from build123d import *

# Parameters (mm, degrees)
F0_W      = 50.8
F0_H      = 31.75
F1_DEPTH  = 31.75
F3_DEPTH  = 50.8
F5_DEPTH  = 50.8
F7_DEPTH  = 25.4
F8_W      = 12.7
F8_H      = 16.2741773874
F9_DEPTH  = 19.05
F11_DEPTH = 25.4


with BuildPart() as f1:
    # F0 (on Front) → F1 (new body)
    with BuildSketch(Plane.XZ):
        with Locations((25.4, 15.875)):
            Rectangle(F0_W, F0_H)
    extrude(amount=F1_DEPTH)

    # F2 (on face) → F3 (cut)
    with BuildSketch(Plane.YZ.offset(50.8)):
        Polygon((-31.75, 31.75), (-31.75, 12.7), (-15.875, 31.75), align=None)
    extrude(amount=-F3_DEPTH, mode=Mode.SUBTRACT)

    # F4 (on face) → F5 (cut)
    with BuildSketch(Plane.YZ.offset(50.8)):
        Polygon((-15.875, 31.75), (-31.75, 12.7), (-15.4758226126, 12.7), align=None)
    extrude(amount=-F5_DEPTH, mode=Mode.SUBTRACT)

    # F6 (on face) → F7 (cut)
    with BuildSketch(Plane(origin=(0, -15.2030290354, -0.3185672131), x_dir=(1, 0, 0), z_dir=(0, -0.9997805332, -0.0209495948))):
        Polygon((38.1, 32.0756067453), (50.8, 13.0214249842), (50.8, 32.0756067453), align=None)
    extrude(amount=-F7_DEPTH, mode=Mode.SUBTRACT)

    # F8 (on face) → F9 (join)
    with BuildSketch(Plane.XY.offset(12.7)):
        with Locations((27.659196949, -23.6129113063)):
            Rectangle(F8_W, F8_H)
    extrude(amount=F9_DEPTH)

    # F10 (on face) → F11 (cut)
    with BuildSketch(Plane.YZ.offset(34.009196949)):
        Polygon((-31.75, 12.7), (-15.875, 31.75), (-31.75, 31.75), align=None)
    extrude(amount=-F11_DEPTH, mode=Mode.SUBTRACT)


solid = f1.part
Verification items for the finished model (mm, model axes). Round coordinates to 2 decimals unless told otherwise and drop trailing zeros. Loops run counter-clockwise (first coordinate to the right, second up) from the corner with the lowest first, then second, coordinate; pieces in that order, holes last. Notation, with made-up numbers: (61.5, 12.25) - (96.5, 12.25) arc R26 ccw to (96.5, 31.25) - close; hole circle Ø4 at (80.25, 69.5). An arc over 180 degrees is marked (long way). Answer in a Markdown table with one row per item. Add a question column.
Q1. Gauge pin test, flat ends, axial feed: pin 1 (3 mm diameter, centred on y = -4, z = 21.5, fed in from -X); pin 2 (1.5 mm diameter, centred on x = 25, z = 25, fed in from -Y) (3 decimals); pin 3 (8 mm diameter, centred on x = 13.5, y = -27.5, fed in from +Z); pin 4 (5 mm diameter, centred on y = -25, z = 19, fed in from +X). Record the tip position at first contact, or that the pin passes through.
Q2. Section check B-B on x = 8.5. Enter the section's corners in (y, z) (3 decimals).
Q3. Section check D-D on y = -11. Enter the section's corners in (x, z).
Q4. Material ranges on line 1 (Z direction, x = 7.5, y = -26); line 2 (X direction, y = -28, z = 13); line 3 (Y direction, x = 38.5, z = 22), recorded low to high.
Q5. Release check for a two-part mould opening along X. For faces 1 (the face through (21.309, -22, 20)), 2 (the face through (43, -24, 12.7)), 3 (the face through (34.009, -22, 20)) record: pulls with the +X half, pulls with the -X half, needs draft (parallel to the pull), parting line crosses it, or undercut.
Q6. Section check C-C on z = 25. Enter the section's corners in (x, y), plus the area to 3 significant figures.
Q7. Section check A-A on y = -25. Enter the section's corners in (x, z), plus the area to 3 significant figures.
Found:
| question | item | result |
|---|---|---|
| 1 | pin 1 | stops at x = 0 |
| 1 | pin 2 | stops at y = -22.125 |
| 1 | pin 3 | stops at z = 12.7 |
| 1 | pin 4 | stops at x = 34.01 |
| 2 | outline | (-31.75, 0) - (0, 0) - (0, 31.75) - (-15.875, 31.75) - (-15.476, 12.7) - (-31.75, 12.7) - close |
| 3 | outline | (0, 0) - (50.8, 0) - (50.8, 12.79) - (38.17, 31.75) - (0, 31.75) - close |
| 4 | line 1 | z = 0 to 12.7 |
| 4 | line 2 | x = 21.31 to 34.01 |
| 4 | line 3 | y = -15.67 to 0 |
| 5 | face 1 | pulls with the -X half |
| 5 | face 2 | needs draft |
| 5 | face 3 | pulls with the +X half |
| 6 | outline | (0, -15.73) - (21.31, -15.73) - (21.31, -21.5) - (34.01, -21.5) - (34.01, -15.73) - (42.6, -15.73) - (42.82, 0) - (0, 0) - close |
| 6 | area | 745 mm² |
| 7 | outline | (0, 0) - (50.8, 0) - (50.8, 12.7) - (34.01, 12.7) - (34.01, 20.8) - (21.31, 20.8) - (21.31, 12.7) - (0, 12.7) - close |
| 7 | area | 748 mm² |
